Job drawing, mm, ordinate dimensions from the low corner. One solid piece. Give positions to 0.01 mm unless a question says otherwise; leave off trailing zeros. Order: outer loops, then holes, each group sorted by start corner. A loop starts at its lowest first (then second) coordinate and runs counter-clockwise, first axis right, second up. Notation, with made-up numbers: (-24, -20.5) -> (-10, -20.5) arc R18 ccw to (-10, 1.5) -> close; hole circle Ø10 at (76.5, 20). An arc over 180 degrees is marked (long way). Use CSV: the item, a comma, the result in double quotes. Start each with the question number.
1. Wall check: line 1 (Z direction, x = 13.75, y = 88.5); line 2 (X direction, y = 10, z = 7.25). Give the ranges that are in metal, low to high. Write a range as from..to.
2. Cut at B-B on z = 4.5. List the corners of the cut face in (x, y).
3. Cut at C-C on y = 45.5. List the corners of the cut face in (x, z), then the cut area to 3 significant figures.
4. Cut at A-A on x = 8. List the corners of the cut face in (y, z), then the cut area to 3 significant figures.
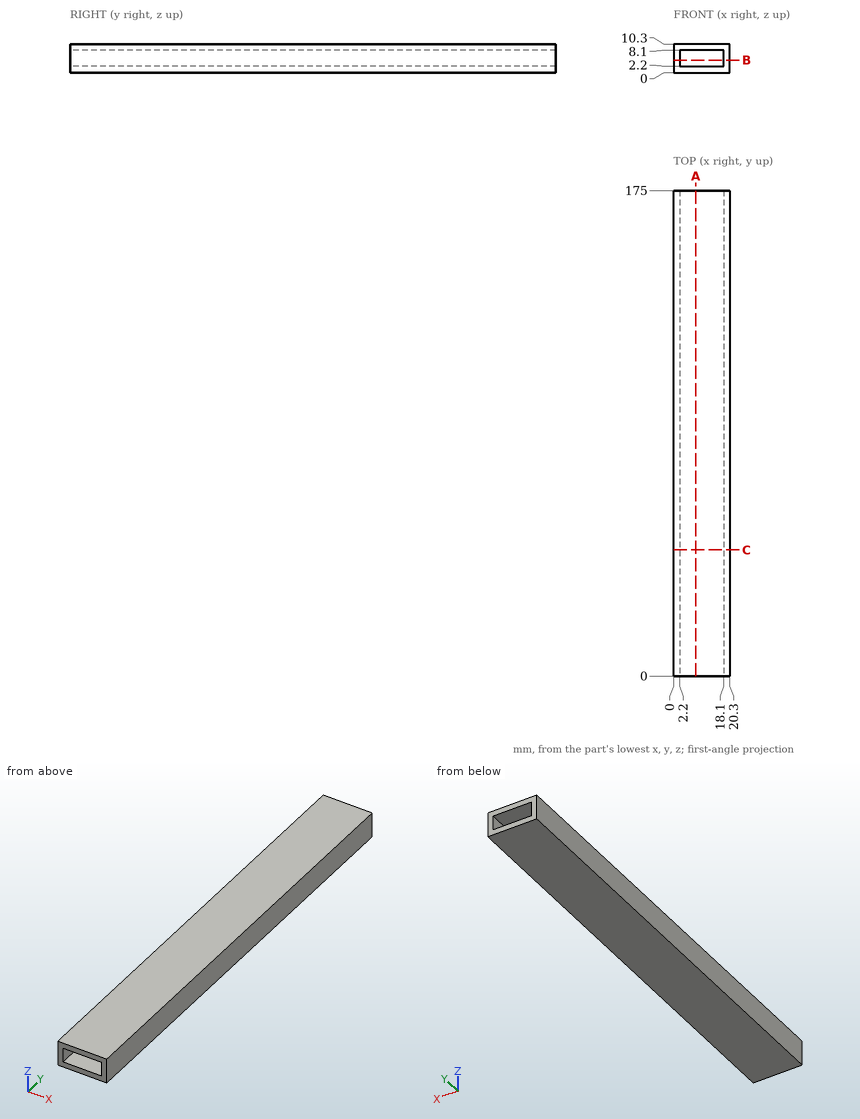
Verdict:
1,line 1,"0..2.2, 8.1..10.3"
1,line 2,"0..2.2, 18.1..20.3"
2,outline,"(0, 0) -> (2.2, 0) -> (2.2, 175) -> (0, 175) -> close; (18.1, 0) -> (20.3, 0) -> (20.3, 175) -> (18.1, 175) -> close"
3,outline,"(0, 0) -> (20.3, 0) -> (20.3, 10.3) -> (0, 10.3) -> close; hole (2.2, 2.2) -> (18.1, 2.2) -> (18.1, 8.1) -> (2.2, 8.1) -> close"
3,area,"115 mm^2"
4,outline,"(0, 0) -> (175, 0) -> (175, 2.2) -> (0, 2.2) -> close; (0, 8.1) -> (175, 8.1) -> (175, 10.3) -> (0, 10.3) -> close"
4,area,"770 mm^2"
